from build123d import *

# Parameters (mm, degrees)
SKETCH1_W           = 31.75
SKETCH1_H           = 26.67
BOSS_EXTRUDE1_DEPTH = 3.175
SKETCH2_R           = 0.95
CUT_EXTRUDE1_DEPTH  = 21.974233597
BOSS_EXTRUDE2_START = 3.175
SKETCH3_R           = 3.175
SKETCH3_R_2         = 0.95
BOSS_EXTRUDE2_DEPTH = 3.175
SKETCH4_W           = 12.7
SKETCH4_H           = 21.59
CUT_EXTRUDE2_DEPTH  = 21.974233597
FILLET1_R           = 2.54
CHAMFER1_SIZE       = 1.27


with BuildPart() as part:
    # Sketch1 → Boss-Extrude1 (new body)
    with BuildSketch(Plane(origin=(0, 0, 0), x_dir=(1, 0, 0), z_dir=(0, 1, 0))):
        Rectangle(SKETCH1_W, SKETCH1_H)
    extrude(amount=BOSS_EXTRUDE1_DEPTH)

    # Sketch2 → Cut-Extrude1 (cut, through all)
    with BuildSketch(Plane(origin=(0, 3.175, 0), x_dir=(1, 0, 0), z_dir=(0, 1, 0))):
        with Locations(Location((-10.795, 7.62, 0), (0, 0, 270))):
            Circle(SKETCH2_R)
        with Locations(Location((10.795, 7.62, 0), (0, 0, 270))):
            Circle(SKETCH2_R)
        with Locations(Location((10.795, -7.62, 0), (0, 0, 270))):
            Circle(SKETCH2_R)
        with Locations(Location((-10.795, -7.62, 0), (0, 0, 270))):
            Circle(SKETCH2_R)
    extrude(amount=-CUT_EXTRUDE1_DEPTH, mode=Mode.SUBTRACT)

    # Sketch3 → Boss-Extrude2 (add)
    # profile 1 of 4: a face of its own
    with BuildSketch(Plane(origin=(0, 3.175, 0), x_dir=(1, 0, 0), z_dir=(0, 1, 0)).offset(BOSS_EXTRUDE2_START)):
        with Locations(Location((-10.795, 7.62, 0), (0, 0, 90))):
            Circle(SKETCH3_R)
        with Locations(Location((-10.795, 7.62, 0), (0, 0, 270))):
            Circle(SKETCH3_R_2, mode=Mode.SUBTRACT)
    # profile 2 of 4: a face of its own
    with BuildSketch(Plane(origin=(0, 3.175, 0), x_dir=(1, 0, 0), z_dir=(0, 1, 0)).offset(BOSS_EXTRUDE2_START)):
        with Locations(Location((10.795, 7.62, 0), (0, 0, 90))):
            Circle(SKETCH3_R)
        with Locations(Location((10.795, 7.62, 0), (0, 0, 270))):
            Circle(SKETCH3_R_2, mode=Mode.SUBTRACT)
    # profile 3 of 4: a face of its own
    with BuildSketch(Plane(origin=(0, 3.175, 0), x_dir=(1, 0, 0), z_dir=(0, 1, 0)).offset(BOSS_EXTRUDE2_START)):
        with Locations(Location((10.795, -7.62, 0), (0, 0, 90))):
            Circle(SKETCH3_R)
        with Locations(Location((10.795, -7.62, 0), (0, 0, 270))):
            Circle(SKETCH3_R_2, mode=Mode.SUBTRACT)
    # profile 4 of 4: a face of its own
    with BuildSketch(Plane(origin=(0, 3.175, 0), x_dir=(1, 0, 0), z_dir=(0, 1, 0)).offset(BOSS_EXTRUDE2_START)):
        with Locations(Location((-10.795, -7.62, 0), (0, 0, 90))):
            Circle(SKETCH3_R)
        with Locations(Location((-10.795, -7.62, 0), (0, 0, 270))):
            Circle(SKETCH3_R_2, mode=Mode.SUBTRACT)
    extrude(amount=-BOSS_EXTRUDE2_DEPTH)

    # Sketch4 → Cut-Extrude2 (cut, through all)
    with BuildSketch(Plane(origin=(0, 3.175, 0), x_dir=(1, 0, 0), z_dir=(0, 1, 0))):
        Rectangle(SKETCH4_W, SKETCH4_H)
    extrude(amount=-CUT_EXTRUDE2_DEPTH, mode=Mode.SUBTRACT)

    # Fillet1
    fillet1_edges = [part.edges().sort_by_distance(p)[0] for p in [
        (6.35, 1.5875, -10.795),
        (6.35, 1.5875, 10.795),
        (-6.35, 1.5875, 10.795),
        (-6.35, 1.5875, -10.795),
        (15.875, 1.5875, 13.335),
        (-15.875, 1.5875, 13.335),
        (-15.875, 1.5875, -13.335),
        (15.875, 1.5875, -13.335),
    ]]
    fillet(fillet1_edges, radius=FILLET1_R)

    # Chamfer1
    chamfer1_edges = [part.edges().sort_by_distance(p)[0] for p in [
        (-10.795, 3.175, -4.445),
        (10.795, 3.175, -4.445),
        (10.795, 3.175, 10.795),
        (-10.795, 3.175, 10.795),
    ]]
    chamfer(chamfer1_edges, length=CHAMFER1_SIZE - 0.0001)  # a hair under: the kernel refuses the full size


solid = part.part
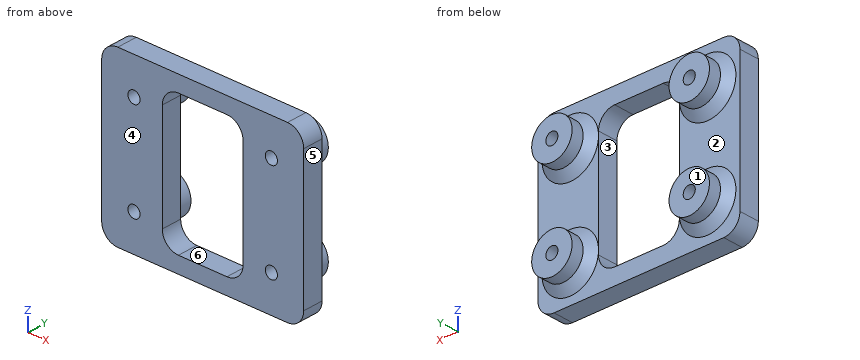
Here's how the part is built. I have some questions about the finished solid (model axes, mm). Face numbers are marked on the shaded views. A direction names the side the tool comes from. Coordinates: 2 decimals unless noted, no trailing zeros. Order: outer loops, then holes, each group sorted by start corner. A loop starts at its lowest first (then second) coordinate and runs counter-clockwise, first axis right, second up. Notation, with made-up numbers: (57.5, -26.5) - (70.5, -26.5) arc R5 ccw to (70.5, -19.5) - close; hole circle Ø11 at (59.25, 49). An arc over 180 degrees is marked (long way). Use CSV: the item, a comma, the result in double quotes. Start each with the question number.
1. If we mould it in two halves opening along X, with no side actions, what happens to the marked faces 4, 5 and 6? For each: +X half, -X half, draft (parallel to the pull), parting line (faces both ways), or undercut.
2. I'm going to push a flat-ended pin straight in: pin 1 (3 mm diameter, centred on x = 9, y = 5.5, fed in from -Z). Where does the tip first touch, or does it pass through?
3. Please list where these lines run through material, in increasing order: line 1 (X direction, y = 2.25, z = 7.62) (3 decimals); line 2 (X direction, y = 4.5, z = -7.62) (3 decimals); line 3 (Z direction, x = -3, y = 1.25) (3 decimals). Write a range as from..to.
4. Suppose I cut it at C-C on x = -1. List the corners of the cut face in (y, z) for me (3 decimals), then the cut area to 3 significant figures.
5. Suppose I cut it at D-D on z = -7.62. Give the number of separate pieces and of enclosed holes in the cut face, then the cut area to 3 significant figures.
6. Suppose I cut it at B-B on y = 6. List the corners of the cut face in (x, z) for me (3 decimals), then the cut area to 3 significant figures.
7. Suppose I cut it at A-A on z = 2.5. List the corners of the cut face in (x, y) for me (3 decimals).
8. For the marked faces 1, 2 and 3, which set-ups out of +Z, -Z, +X, -X, +Y, -Y let a thin tool reach every point of the face, with its end or its side?
Output:
1,face 4,"draft"
1,face 5,"+X half"
1,face 6,"undercut"
2,pin 1,"stops at z = -10.91"
3,line 1,"x = -15.875..-11.745, -9.845..-6.35, 6.35..9.845, 11.745..15.875"
3,line 2,"x = -13.97..-11.745, -9.845..-7.62, 7.62..9.845, 11.745..13.97"
3,line 3,"z = -13.335..-10.795, 10.795..13.335"
4,outline,"(0, -13.335) - (3.175, -13.335) - (3.175, -10.795) - (0, -10.795) - close; (0, 10.795) - (3.175, 10.795) - (3.175, 13.335) - (0, 13.335) - close"
4,area,"16.1 mm2"
5,separate pieces,"4"
5,enclosed holes,"0"
5,area,"79.9 mm2"
6,outline,"circle Ø6.35 at (-10.795, -7.62); circle Ø6.35 at (-10.795, 7.62); circle Ø6.35 at (10.795, -7.62); circle Ø6.35 at (10.795, 7.62); hole circle Ø1.9 at (-10.795, -7.62); hole circle Ø1.9 at (-10.795, 7.62); hole circle Ø1.9 at (10.795, -7.62); hole circle Ø1.9 at (10.795, 7.62)"
6,area,"115 mm2"
7,outline,"(-15.875, 0) - (-6.35, 0) - (-6.35, 3.175) - (-15.875, 3.175) - close; (6.35, 0) - (15.875, 0) - (15.875, 3.175) - (6.35, 3.175) - close"
8,face 1,"+Z, -Z, +X, -X, +Y"
8,face 2,"+Y"
8,face 3,"+Y, -Y"
